For this review, take the finished solid that the model builds, in its own axes (mm). A direction names the side the tool comes from. Round coordinates to 2 decimals unless told otherwise and drop trailing zeros. Loops run counter-clockwise (first coordinate to the right, second up) from the corner with the lowest first, then second, coordinate; pieces in that order, holes last.
1) Take a section at B-B (y = 410). State the section outline as (x, z) points, then the cut area to 3 significant figures.
2) Take a section at D-D (x = 567.5). State the section outline as (y, z) points.
3) Take a section at A-A (y = 650). State the section outline as (x, z) points, then the cut area to 3 significant figures.
4) Tool access review of faces 5 (the flat face through (471, 100, 49)), 6 (the cylindrical face through (251.21, 184.964, 14.258)), 7 (the cylindrical face through (251.21, 155.42, 25.594)), 8 (the flat face through (750, 651, 1931)): name each direction out of +Z, -Z, +X, -X, +Y, -Y from which nothing blocks a thin tool from reaching the whole face with its end or side.
5) Take a section at C-C (z = 794). State the section outline as (x, y) points.
6) Mouldability with a two-part tool opening along Y and no side actions: class faces 1 (the flat face through (-286.7, 127.1, 60.4)), 2 (the flat face through (10, 94, 0)), 3 (the flat face through (216.7, 127.1, 60.4)), 4 (the flat face through (10, 0, 49)) as pulls with the +Y half, pulls with the -Y half, needs draft (parallel to the pull), parting line crosses it, or undercut.
7) Wall thickness on L1, parallel to Y at x = -193, z = 83; L2, parallel to Y at x = -760, z = 1960; L3, parallel to Z at x = 717, y = 67: over which ranges is each line inside the solid? List them lowest first.
```python
from build123d import *

# Parameters (mm, degrees)
SALIENTE_EXTRUIR1_DEPTH = 750
CORTAR_EXTRUIR4_REACH   = 2536.265
CROQUIS3_W              = 1300
CROQUIS3_H              = 1300
CORTAR_EXTRUIR5_REACH   = 2536.265
CROQUIS4_W              = 1300
CROQUIS4_H              = 504.649156168
CROQUIS5_R              = 27.184697772
SALIENTE_EXTRUIR2_DEPTH = 50
SALIENTE_EXTRUIR3_DEPTH = 100
CROQUIS8_R              = 27.1845
SALIENTE_EXTRUIR4_DEPTH = 50
SALIENTE_EXTRUIR5_DEPTH = 100
CROQUIS11_W             = 70
CROQUIS11_H             = 100
SALIENTE_EXTRUIR6_DEPTH = 100
REDONDEO1_R             = 50
CORTAR_EXTRUIR6_REACH   = 2735.316
CROQUIS12_R             = 25


with BuildPart() as part:
    # Croquis1 → Saliente-Extruir1 (new, symmetric)
    with BuildSketch(Plane(origin=(0, 0, 0), x_dir=(0, 0, -1), z_dir=(1, 0, 0))):
        Polygon((-100, 700), (-100, 1500), (0, 1500), (0, 0), (-100, 0), (-100, 600), (-1800, 600), (-1800, 0), (-1900, 0), (-1900, 600), (-1900, 700), align=None)
    extrude(amount=SALIENTE_EXTRUIR1_DEPTH, both=True)

    # Cortar-Extruir4: up to this face of the body (flat: up to its plane)
    cortar_extruir4_end = Plane(part.part.faces().sort_by_distance((0, 300, 1800))[0])
    # Croquis3 → Cortar-Extruir4 (cut, up to the picked face)
    with BuildSketch(Plane(origin=(0, 0, 0), x_dir=(-1, 0, 0), z_dir=(0, 0, -1)), mode=Mode.PRIVATE) as cortar_extruir4_sk1:
        with Locations((0, 750)):
            Rectangle(CROQUIS3_W, CROQUIS3_H)
    cortar_extruir4_tool1 = split(extrude(cortar_extruir4_sk1.sketch, amount=-CORTAR_EXTRUIR4_REACH, mode=Mode.PRIVATE), bisect_by=cortar_extruir4_end, keep=Keep.BOTH, mode=Mode.PRIVATE)
    add(cortar_extruir4_tool1.solids().sort_by(Axis((0, 750, 0), (0, 0, 1)))[0], mode=Mode.SUBTRACT)

    # Croquis4 → Cortar-Extruir5 (cut, up to next)
    with BuildSketch(Plane.XY.offset(1900), mode=Mode.PRIVATE) as cortar_extruir5_sk1:
        with Locations((0, 352.324578084)):
            Rectangle(CROQUIS4_W, CROQUIS4_H)
    cortar_extruir5_tool1 = extrude(cortar_extruir5_sk1.sketch, amount=-CORTAR_EXTRUIR5_REACH, mode=Mode.PRIVATE) & part.part
    add(cortar_extruir5_tool1.solids().sort_by_distance((0, 352.324578, 1900))[0], mode=Mode.SUBTRACT)



with BuildPart() as body_2:
    # Croquis5 → Saliente-Extruir2 (new body)
    with BuildSketch(Plane(origin=(750, 0, 0), x_dir=(0, 0, -1), z_dir=(1, 0, 0))):
        with BuildLine():
            Line((-1960, 600), (-1900, 600))
            Line((-1900, 600), (-1900, 700))
            Line((-1900, 700), (-1960, 700))
            ThreePointArc((-1960, 700), (-2010, 650), (-1960, 600))
        make_face()
        with Locations((-1960, 650)):
            Circle(CROQUIS5_R, mode=Mode.SUBTRACT)
    extrude(amount=SALIENTE_EXTRUIR2_DEPTH)


with BuildPart() as part_1:
    add(part.part)

    add(body_2.part)  # Saliente-Extruir3 merges body 2
    # Croquis6 → Saliente-Extruir3 (add)
    with BuildSketch(Plane(origin=(0, 700, 0), x_dir=(1, 0, 0), z_dir=(0, 1, 0))):
        Polygon((750, -1900), (800, -1900), (750, -1762.626129027), align=None)
    extrude(amount=-SALIENTE_EXTRUIR3_DEPTH)



with BuildPart() as body_2_2:
    # Croquis8 → Saliente-Extruir4 (new body)
    with BuildSketch(Plane.ZY.offset(750)):
        with BuildLine():
            Line((1960, 700), (1900, 700))
            Line((1900, 700), (1900, 600))
            Line((1900, 600), (1960, 600))
            ThreePointArc((1960, 600), (2010, 650), (1960, 700))
        make_face()
        with Locations((1960, 650)):
            Circle(CROQUIS8_R, mode=Mode.SUBTRACT)
    extrude(amount=SALIENTE_EXTRUIR4_DEPTH)


with BuildPart() as part_2:
    add(part_1.part)

    add(body_2_2.part)  # Saliente-Extruir5 merges body 2 2
    # Croquis9 → Saliente-Extruir5 (add)
    with BuildSketch(Plane(origin=(0, 700, 0), x_dir=(1, 0, 0), z_dir=(0, 1, 0))):
        Polygon((-750, -1900), (-800, -1900), (-750, -1762.626129027), align=None)
    extrude(amount=-SALIENTE_EXTRUIR5_DEPTH)

    # Croquis11 → Saliente-Extruir6 (add)
    with BuildSketch(Plane(origin=(0, 0, 0), x_dir=(-1, 0, 0), z_dir=(0, 0, -1))):
        with Locations((-251.7, 150)):
            Rectangle(CROQUIS11_W, CROQUIS11_H)
        with Locations((251.7, 150)):
            Rectangle(CROQUIS11_W, CROQUIS11_H)
    extrude(amount=-SALIENTE_EXTRUIR6_DEPTH)

    # Redondeo1
    redondeo1_edges = [part_2.edges().sort_by_distance(p)[0] for p in [
        (251.7, 200, 100),
        (251.7, 200, 0),
        (-251.7, 200, 100),
        (-251.7, 200, 0),
    ]]
    fillet(redondeo1_edges, radius=REDONDEO1_R - 0.0001)  # a hair under: the kernel refuses the full size

    # Cortar-Extruir6: up to this face of the body (flat: up to its plane)
    cortar_extruir6_end = Plane(part_2.part.faces().sort_by_distance((286.7, 145.332525283, 50))[0])
    # Croquis12 → Cortar-Extruir6 (cut, up to the picked face)
    with BuildSketch(Plane.ZY.offset(286.7), mode=Mode.PRIVATE) as cortar_extruir6_sk1:
        with Locations(Location((50, 150, 0), (0, 0, 270))):
            Circle(CROQUIS12_R)
    cortar_extruir6_tool1 = split(extrude(cortar_extruir6_sk1.sketch, amount=-CORTAR_EXTRUIR6_REACH, mode=Mode.PRIVATE), bisect_by=cortar_extruir6_end, keep=Keep.BOTH, mode=Mode.PRIVATE)
    add(cortar_extruir6_tool1.solids().sort_by(Axis((-286.7, 150, 50), (1, 0, 0)))[0], mode=Mode.SUBTRACT)


solid = part_2.part
```
Response:
1. outline: (-750, 0) - (-650, 0) - (-650, 100) - (-750, 100) - close; (-750, 1800) - (-650, 1800) - (-650, 1900) - (-750, 1900) - close; (650, 0) - (750, 0) - (750, 100) - (650, 100) - close; (650, 1800) - (750, 1800) - (750, 1900) - (650, 1900) - close
1. area: 40,000 mm2
2. outline: (0, 0) - (100, 0) - (100, 100) - (0, 100) - close; (0, 1800) - (100, 1800) - (100, 1900) - (0, 1900) - close; (604.65, 1800) - (700, 1800) - (700, 1900) - (604.65, 1900) - close; (1400, 0) - (1500, 0) - (1500, 100) - (1400, 100) - close
3. outline: (-800, 1900) - (-750, 1762.63) - (-750, 0) - (-650, 0) - (-650, 1800) - (650, 1800) - (650, 0) - (750, 0) - (750, 1762.63) - (800, 1900) - (800, 1932.82) - (750, 1932.82) - (750, 1900) - (-750, 1900) - (-750, 1932.82) - (-800, 1932.82) - close; (-800, 1987.18) - (-750, 1987.18) - (-750, 2010) - (-800, 2010) - close; (750, 1987.18) - (800, 1987.18) - (800, 2010) - (750, 2010) - close
3. area: 522,000 mm2
4. face 5: +Z, -Z
4. face 6: -Z
4. face 7: none
4. face 8: +Z, +Y, -Y
5. outline: (-750, 600) - (-650, 600) - (-650, 700) - (-750, 700) - close; (650, 600) - (750, 600) - (750, 700) - (650, 700) - close
6. face 1: undercut
6. face 2: needs draft
6. face 3: undercut
6. face 4: pulls with the -Y half
7. L1: y = 0 to 100, 1400 to 1500
7. L2: y = 600 to 622.82, 677.18 to 700
7. L3: z = 0 to 100, 1800 to 1900
